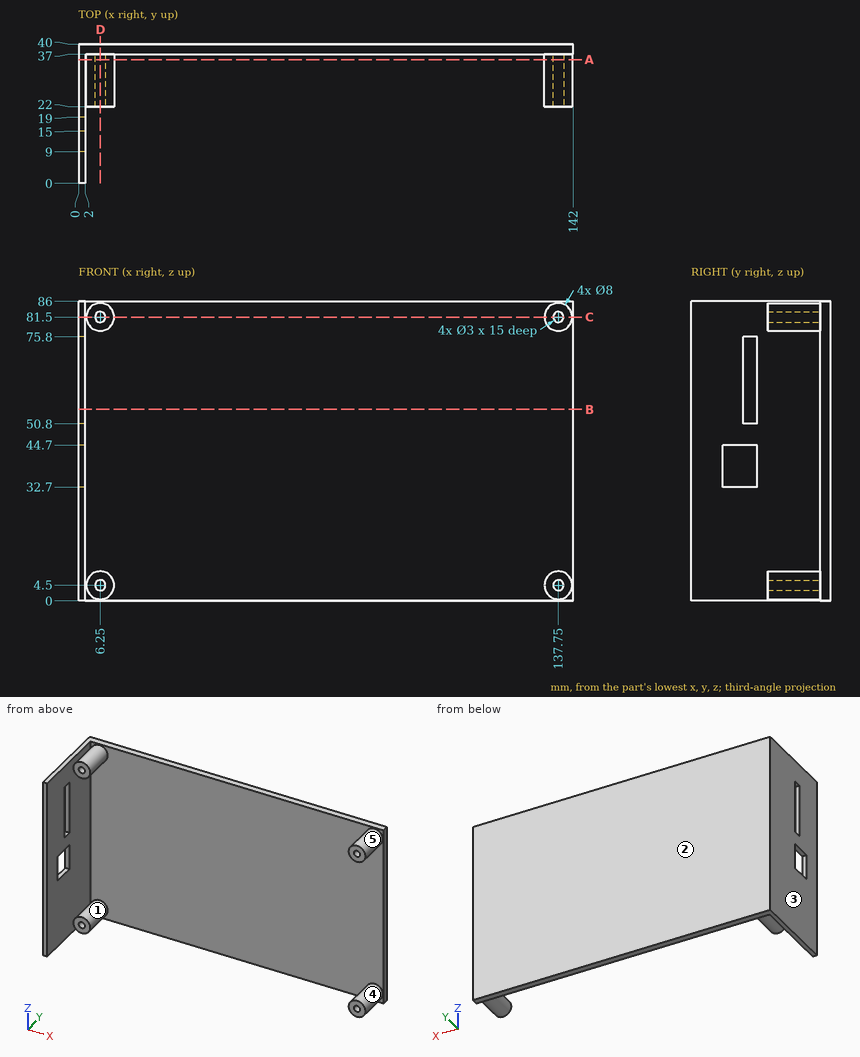
Part print with two shaded views. Sizes in mm from the minimum x, y, z corner. A direction names the side the tool comes from. Round coordinates to 2 decimals unless told otherwise and drop trailing zeros. Order: outer loops, then holes, each group sorted by start corner. A loop starts at its lowest first (then second) coordinate and runs counter-clockwise, first axis right, second up. Notation, with made-up numbers: M 49.5,10.5 L 108.5,10.5 A23 ccw 108.5,20.5 Z; hole C -17,72 d6. An arc over 180 degrees is marked long. Put each result on its own line as item: value. Start each with the question number.
1. Drill centre lines: probe 1 along Z at (x, y) = (6, 33); probe 2 along X at (y, z) = (30, 81); probe 3 along X at (y, z) = (19, 17). Where is each one in solid material? Low to high. Write a range as [from, to].
2. Drop flat-ended pins along their axis: pin 1 (1 mm diameter, centred on y = 8.5, z = 14.5, fed in from +X); pin 2 (2.5 mm diameter, centred on x = 8, z = 3.5, fed in from -Y); pin 3 (2.5 mm diameter, centred on x = 137.75, z = 4.5, fed in from -Y). Give the stop position or say it passes through.
3. Slice it at A-A on y = 35.5. State how many separate pieces and enclosed holes the cut face has, then the cut area to 3 significant figures.
4. Two-plate mould, pull along Z, no slides. Class the marked faces 3, 4 and 5: +Z half, -Z half, draft (parallel to the pull), parting line (faces both ways), or undercut.
5. Slice it at B-B on z = 55. List the corners of the cut face in (x, y), then the cut area to 3 significant figures.
6. Slice it at C-C on z = 81.5. List the corners of the cut face in (x, y), then the cut area to 3 significant figures.
7. Tool access for the marked faces 1 and 2: list every direction of +Z, -Z, +X, -X, +Y, -Y with a clear straight run to the whole face (end or side of a thin tool).
8. Slice it at D-D on x = 6.25. List the corners of the cut face in (y, z), then the cut area to 3 significant figures.
Findings:
1. probe 1: [0.51, 3.02], [5.98, 8.49], [77.51, 80.02], [82.98, 85.49]
1. probe 2: [0, 2], [2.28, 4.84], [7.66, 10.22], [133.78, 136.34], [139.16, 141.72]
1. probe 3: [0, 2]
2. pin 1: x = 2
2. pin 2: y = 22
2. pin 3: y = 37
3. separate pieces: 5
3. enclosed holes: 4
3. area: 345 mm2
4. face 3: draft
4. face 4: undercut
4. face 5: undercut
5. outline: M 0,0 L 2,0 L 2,15 L 0,15 Z; M 0,19 L 2,19 L 2,37 L 142,37 L 142,40 L 0,40 Z
5. area: 492 mm2
6. outline: M 0,0 L 2,0 L 2,37 L 2.25,37 L 2.25,22 L 4.75,22 L 4.75,37 L 7.75,37 L 7.75,22 L 10.25,22 L 10.25,37 L 133.75,37 L 133.75,22 L 136.25,22 L 136.25,37 L 139.25,37 L 139.25,22 L 141.75,22 L 141.75,37 L 142,37 L 142,40 L 0,40 Z
6. area: 650 mm2
7. face 1: -Y
7. face 2: +Z, -Z, +X, -X, +Y
8. outline: M 22,0.5 L 37,0.5 L 37,0 L 40,0 L 40,86 L 37,86 L 37,85.5 L 22,85.5 L 22,83 L 37,83 L 37,80 L 22,80 L 22,77.5 L 37,77.5 L 37,8.5 L 22,8.5 L 22,6 L 37,6 L 37,3 L 22,3 Z
8. area: 408 mm2
